Geometry: see drawing. Coordinates: mm, zero at the bounding-box minimum. A direction names the side the tool comes from. Round coordinates to 2 decimals unless told otherwise and drop trailing zeros. Write each loop counter-clockwise with the first axis right and the second up, starting at its lowest first coordinate (ties: lowest second). Pieces come first, ordered by that corner, then holes. Notation, with made-up numbers: (1.5, 9) -> (16.5, 9) arc R23 cw to (16.5, 26) -> close; hole circle Ø10 at (38, 36). An arc over 180 degrees is marked (long way). Use CSV: the item, a comma, the result in double quotes.
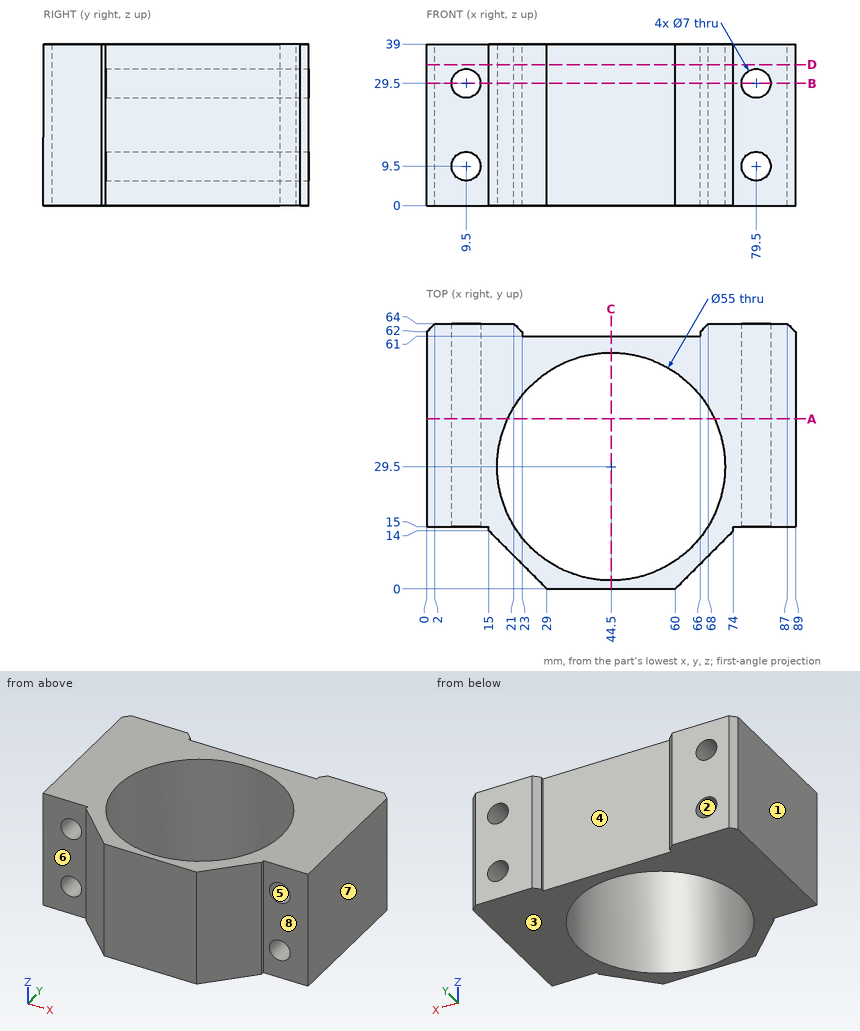
Item 1: Set-up query: the marked faces 4, 5, 6, 7 and 8. Return all of +Z, -Z, +X, -X, +Y, -Y with unobstructed straight access to the full face (end or side cutting, diameter ignored); none if empty.
Worked answers:
face 4,"+Z, -Z, +Y"
face 5,"+Y, -Y"
face 6,"+Z, -Z, -X, -Y"
face 7,"+Z, -Z, +X, +Y, -Y"
face 8,"+Z, -Z, +X, -Y"
Item 2: Section query B-B on z = 29.5. Return the cut outline in (x, y).
Worked answers:
outline,"(0, 15) -> (6, 15) -> (6, 64) -> (2, 64) -> (0, 62) -> close; (13, 15) -> (15, 15) -> (15, 14) -> (29, 0) -> (60, 0) -> (74, 14) -> (74, 15) -> (76, 15) -> (76, 64) -> (68, 64) -> (66, 62) -> (66, 61) -> (23, 61) -> (23, 62) -> (21, 64) -> (13, 64) -> close; (83, 15) -> (89, 15) -> (89, 62) -> (87, 64) -> (83, 64) -> close; hole circle Ø55 at (44.5, 29.5)"
Item 3: Section query A-A on y = 41. Return the cut outline in (x, z), plus the area to 3 significant figures.
Worked answers:
outline,"(0, 0) -> (19.52, 0) -> (19.52, 39) -> (0, 39) -> close; (69.48, 0) -> (89, 0) -> (89, 39) -> (69.48, 39) -> close; hole circle Ø7 at (9.5, 9.5); hole circle Ø7 at (9.5, 29.5); hole circle Ø7 at (79.5, 9.5); hole circle Ø7 at (79.5, 29.5)"
area,"1,370 mm²"
Item 4: Line query: line 1 (Z direction, x = 9.5, y = 30.5); line 2 (X direction, y = 43.5, z = 27); line 3 (X direction, y = 29.5, z = 14). Output: solid intervals per line, ascending.
Worked answers:
line 1,"z = 0 to 6, 13 to 26, 33 to 39"
line 2,"x = 0 to 7.05, 11.95 to 20.83, 68.17 to 77.05, 81.95 to 89"
line 3,"x = 0 to 17, 72 to 89"
Item 5: First-contact query: pin 1 Ø16.5 at (x, z) = (80, 16.5) entering from -Y; pin 2 Ø6 at (x, z) = (27.5, 21.5) entering from -Y; pin 3 Ø4 at (x, z) = (21.5, 32) entering from -Y; pin 4 Ø0.8 at (y, z) = (14.5, 13.5) entering from +X. Flat tips, straight axial feed; report the tip coordinate or a pass-through.
Worked answers:
pin 1,"stops at y = 11.75"
pin 2,"stops at y = 0"
pin 3,"stops at y = 5.5"
pin 4,"stops at x = 74"
Item 6: Pull-direction query (X, two-part tool) for the marked faces 1, 2 and 3; classes: +X half, -X half, draft (parallel to the pull), parting line (faces both ways), or undercut.
Worked answers:
face 1,"-X half"
face 2,"undercut"
face 3,"draft"
Item 7: Section query D-D on z = 34. Return the cut outline in (x, y).
Worked answers:
outline,"(0, 15) -> (15, 15) -> (15, 14) -> (29, 0) -> (60, 0) -> (74, 14) -> (74, 15) -> (89, 15) -> (89, 62) -> (87, 64) -> (68, 64) -> (66, 62) -> (66, 61) -> (23, 61) -> (23, 62) -> (21, 64) -> (2, 64) -> (0, 62) -> close; hole circle Ø55 at (44.5, 29.5)"
Item 8: Section query C-C on x = 44.5. Return the cut outline in (y, z).
Worked answers:
outline,"(0, 0) -> (2, 0) -> (2, 39) -> (0, 39) -> close; (57, 0) -> (61, 0) -> (61, 39) -> (57, 39) -> close"
